Check sheet for the drawn part. Datum: minimum x, y, z corner. Units: mm. A direction names the side the tool comes from. Round coordinates to 2 decimals unless told otherwise and drop trailing zeros. Order: outer loops, then holes, each group sorted by start corner. A loop starts at its lowest first (then second) coordinate and runs counter-clockwise, first axis right, second up. Notation, with made-up numbers: (44, 66.25) -> (100, 66.25) arc R19 ccw to (100, 71.25) -> close; hole circle Ø5 at (81, 66.5). An arc over 180 degrees is marked (long way). Answer in a Markdown table with one row per item.
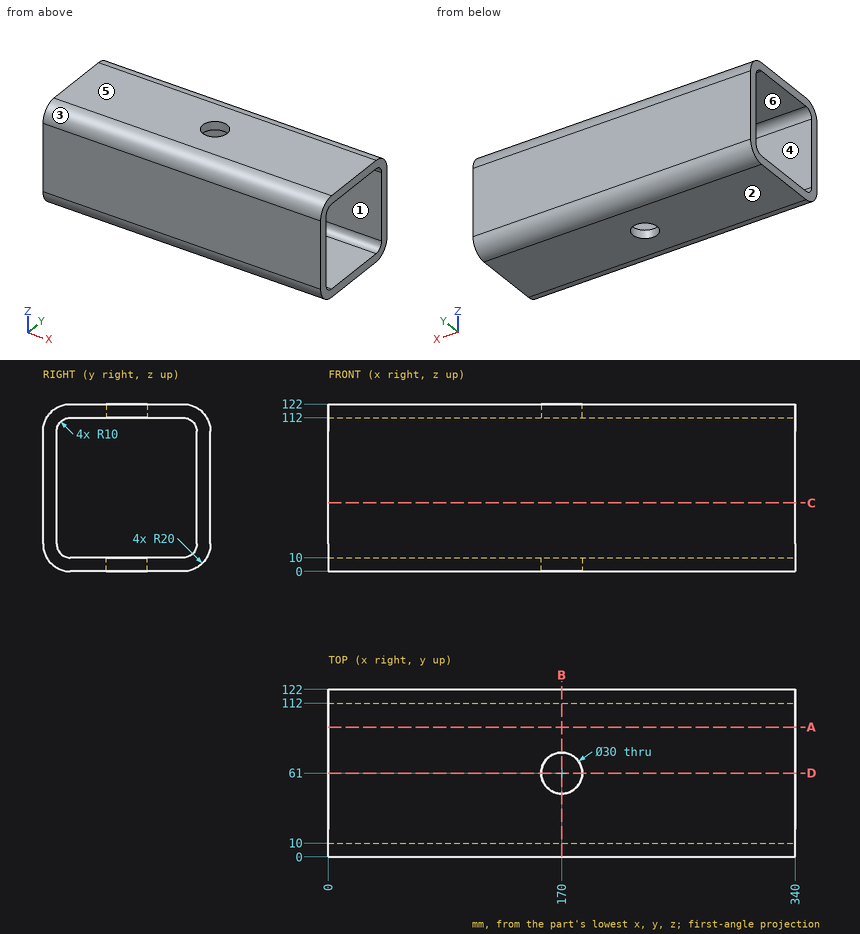
(1) Scan lines: probe 1 along Y at (x, z) = (110, 24); probe 2 along X at (y, z) = (61, 115). Record each from-to range of solid material in increasing order. Write a range as from..to.
Solutions:
| item | result |
|---|---|
| probe 1 | 0..10, 112..122 |
| probe 2 | 0..155, 185..340 |
(2) Section check B-B on x = 170. Record the boundary of the cut face in (y, z), plus the area to 3 significant figures.
Solutions:
| item | result |
|---|---|
| outline | (0, 20) arc R20 ccw to (20, 0) -> (46, 0) -> (46, 10) -> (20, 10) arc R10 cw to (10, 20) -> (10, 102) arc R10 cw to (20, 112) -> (46, 112) -> (46, 122) -> (20, 122) arc R20 ccw to (0, 102) -> close; (76, 0) -> (102, 0) arc R20 ccw to (122, 20) -> (122, 102) arc R20 ccw to (102, 122) -> (76, 122) -> (76, 112) -> (102, 112) arc R10 cw to (112, 102) -> (112, 20) arc R10 cw to (102, 10) -> (76, 10) -> close |
| area | 3,620 mm^2 |
(3) Draft check along Y on the marked faces 3, 4, 5 and 6. Enter one of: pulls with the +Y half, pulls with the -Y half, needs draft (parallel to the pull), parting line crosses it, or undercut.
Solutions:
| item | result |
|---|---|
| face 3 | pulls with the -Y half |
| face 4 | undercut |
| face 5 | needs draft |
| face 6 | undercut |
(4) Section check A-A on y = 94.5. Record the boundary of the cut face in (x, z).
Solutions:
| item | result |
|---|---|
| outline | (0, 0) -> (340, 0) -> (340, 10) -> (0, 10) -> close; (0, 112) -> (340, 112) -> (340, 122) -> (0, 122) -> close |
(5) Section check D-D on y = 61. Record the boundary of the cut face in (x, z), plus the area to 3 significant figures.
Solutions:
| item | result |
|---|---|
| outline | (0, 0) -> (155, 0) -> (155, 10) -> (0, 10) -> close; (0, 112) -> (155, 112) -> (155, 122) -> (0, 122) -> close; (185, 0) -> (340, 0) -> (340, 10) -> (185, 10) -> close; (185, 112) -> (340, 112) -> (340, 122) -> (185, 122) -> close |
| area | 6,200 mm^2 |
(6) Tool access check on the marked faces 1 and 2. Record the directions out of +Z, -Z, +X, -X, +Y, -Y that give a thin tool (end or side, any length) a straight path to the whole face; none if there is none.
Solutions:
| item | result |
|---|---|
| face 1 | +X, -X |
| face 2 | -Z, +X, -X, +Y, -Y |
(7) Depth check by flat-ended pin: pin 1 Ø1 at (x, z) = (250, 40) entering from -Y; pin 2 Ø5 at (y, z) = (74.5, 107.5) entering from -X. Enter the tip coordinate at first touch or a pass-through.
Solutions:
| item | result |
|---|---|
| pin 1 | y = 0 |
| pin 2 | through |
